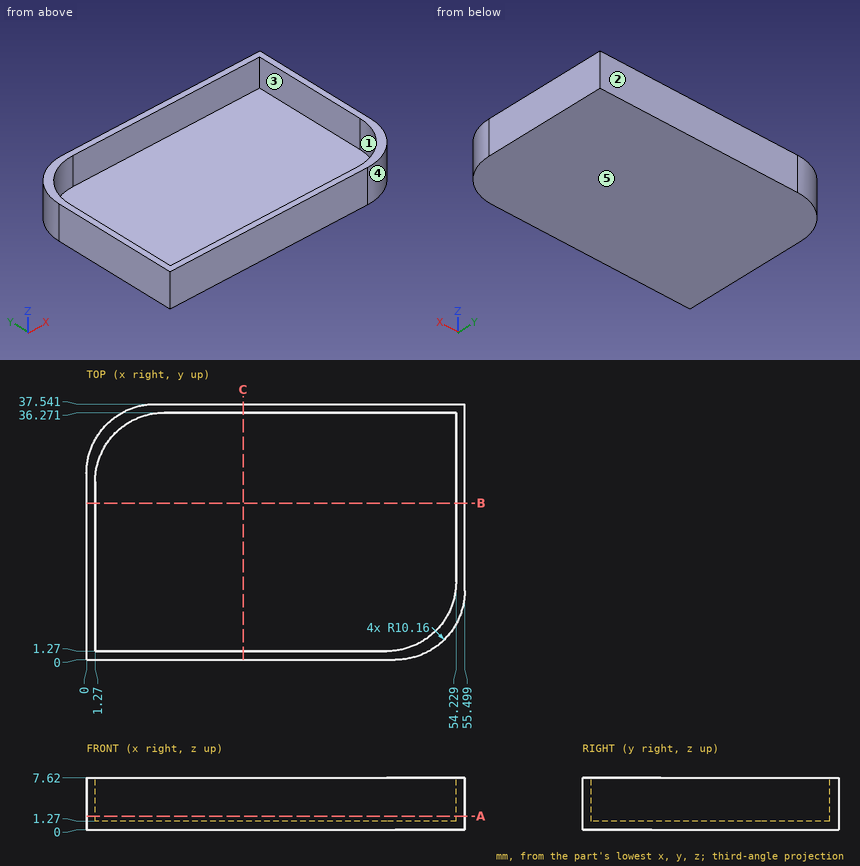
Geometry check sheet. Reference: drawing and pictorial views, mm from the part's lowest x, y, z. A direction names the side the tool comes from. Give positions to 0.01 mm unless a question says otherwise; leave off trailing zeros. Loops run counter-clockwise (first coordinate to the right, second up) from the corner with the lowest first, then second, coordinate; pieces in that order, holes last. Notation, with made-up numbers: (4, 55) -> (42, 55) arc R21 cw to (42, 88) -> close; hole circle Ø9 at (-39.5, 58). An arc over 180 degrees is marked (long way). Answer in a Markdown table with one row per item. Add a question column.
1) Gauge pin test, flat end, axial feed: P1, Ø1.5, axis at x = 13.5, y = 13, coming from the +Z side. Record the tip position at first contact, or that the pin passes through.
2) Set-up check for the marked faces 1 and 2: record each of +Z, -Z, +X, -X, +Y, -Y from which the full face is reachable in a straight line by a thin tool's end or side.
3) Material ranges on probe 1 along Y at (x, z) = (21.5, 2.5); probe 2 along X at (y, z) = (24, 4.75); probe 3 along Z at (x, y) = (53.5, 27), recorded low to high. Write a range as from..to.
4) Cross-section at A-A on z = 2. Record the boundary of the cut face in (x, y).
5) Cross-section at B-B on y = 23. Record the boundary of the cut face in (x, z).
6) Cross-section at C-C on x = 23. Record the boundary of the cut face in (y, z).
7) Draft check along X on the marked faces 3, 4 and 5. Enter one of: pulls with the +X half, pulls with the -X half, needs draft (parallel to the pull), parting line crosses it, or undercut.
Outcome:
| question | item | result |
|---|---|---|
| 1 | P1 | stops at z = 1.27 |
| 2 | face 1 | +Z |
| 2 | face 2 | +Z, -Z, +X, -X, +Y |
| 3 | probe 1 | y = 0..1.27, 36.27..37.54 |
| 3 | probe 2 | x = 0..1.27, 54.23..55.5 |
| 3 | probe 3 | z = 0..1.27 |
| 4 | outline | (0, 0) -> (45.34, 0) arc R10.16 ccw to (55.5, 10.16) -> (55.5, 37.54) -> (10.16, 37.54) arc R10.16 ccw to (0, 27.38) -> close; hole (1.27, 1.27) -> (44.07, 1.27) arc R10.16 ccw to (54.23, 11.43) -> (54.23, 36.27) -> (11.43, 36.27) arc R10.16 ccw to (1.27, 26.11) -> close |
| 5 | outline | (0, 0) -> (55.5, 0) -> (55.5, 7.62) -> (54.23, 7.62) -> (54.23, 1.27) -> (1.27, 1.27) -> (1.27, 7.62) -> (0, 7.62) -> close |
| 6 | outline | (0, 0) -> (37.54, 0) -> (37.54, 7.62) -> (36.27, 7.62) -> (36.27, 1.27) -> (1.27, 1.27) -> (1.27, 7.62) -> (0, 7.62) -> close |
| 7 | face 3 | undercut |
| 7 | face 4 | pulls with the +X half |
| 7 | face 5 | needs draft |
